from build123d import *

# Parameters (mm, degrees)
F0_W      = 82.55
F0_H      = 82.55
F1_DEPTH  = 38.1
F2_W      = 82.55
F2_H      = 82.55
F2_W_2    = 13.9428069815
F2_H_2    = 9.9208420143
F2_W_3    = 8.0439243466
F2_H_3    = 6.4351418987
F2_W_4    = 8.2115095574
F2_H_4    = 6.1912699603
F2_W_5    = 5.6307478808
F2_H_5    = 5.2285513375
F2_W_6    = 10.3230390232
F2_H_6    = 9.3845799565
F2_W_7    = 7.6417308301
F2_H_7    = 7.5076650828
F2_W_8    = 12.3340208083
F2_H_8    = 10.3230387904
F2_W_9    = 7.9098585993
F2_H_9    = 7.5076660141
F2_W_10   = 7.2456169873
F2_H_10   = 6.6790115088
F2_W_11   = 6.5692057833
F2_H_11   = 4.9604205415
F2_W_12   = 14.4120394252
F2_H_12   = 10.4571059346
F2_W_13   = 11.3955624402
F2_H_13   = 10.1889744401
F2_W_14   = 6.7032724619
F2_H_14   = 5.6307483464
F2_W_15   = 5.6307520717
F2_H_15   = 5.3626168519
F3_DEPTH  = 2.54
F4_W      = 82.55
F4_H      = 12.5048903072
F5_DEPTH  = 2.286
F6_W      = 8.554907316
F6_H      = 8.3226170391
F7_DEPTH  = 2.286
F8_W      = 8.5991304368
F8_H      = 7.9995281994
F9_DEPTH  = 2.286
F10_W     = 9.0507952429
F10_H     = 8.4728021175
F11_DEPTH = 2.286
F12_W     = 7.5796225905
F12_H     = 8.1127006561
F13_DEPTH = 2.286
F14_W     = 84.836
F14_H     = 12.5993990594
F15_DEPTH = 2.286
F16_W     = 5.275822799
F16_H     = 8.0181919038
F17_DEPTH = 2.286
F18_W     = 2.1420419216
F18_H     = 8.0181919038
F19_DEPTH = 2.286
F20_W     = 9.7789997235
F20_H     = 7.7714007348
F21_DEPTH = 2.286
F22_W     = 8.092913311
F22_H     = 7.8396778554
F23_DEPTH = 2.286
F24_W     = 7.9482773185
F24_H     = 8.0201905221
F25_DEPTH = 2.286
F26_W     = 84.836
F26_H     = 12.4227774584
F27_DEPTH = 2.286
F28_W     = 5.6573223279
F28_H     = 8.1968121231
F29_DEPTH = 2.286
F30_W     = 2.7038902044
F30_H     = 8.1968121231
F31_DEPTH = 2.286
F32_W     = 11.1818928272
F32_H     = 7.734913379
F33_DEPTH = 2.286
F34_W     = 11.2993712537
F34_H     = 7.8291036189
F35_DEPTH = 2.286
F36_W     = 7.6127404213
F36_H     = 7.734913379
F37_DEPTH = 2.286
F38_W     = 87.122
F38_H     = 10.4137536731
F39_DEPTH = 2.286
F40_W     = 4.9288716123
F40_H     = 9.7913470712
F40_W_2   = 2.5759153068
F41_DEPTH = 2.286
F42_W     = 11.5772541612
F42_H     = 9.7913470712
F43_DEPTH = 2.286
F44_W     = 13.4015749209
F44_H     = 9.7913470712
F45_DEPTH = 2.286
F46_W     = 7.5191628144
F46_H     = 10.4137536731
F47_DEPTH = 2.286
F48_SCALE = 1.5


with BuildPart() as f1:
    # F0 (on Top) → F1 (new body)
    with BuildSketch(Plane.XY):
        Rectangle(F0_W, F0_H)
    extrude(amount=F1_DEPTH)

    # F2 (on face) → F3 (join)
    with BuildSketch(Plane.XY.offset(38.1)):
        Rectangle(F2_W, F2_H)
        with Locations((-21.3224873878, -29.7867883928)):
            Rectangle(F2_W_2, F2_H_2, mode=Mode.SUBTRACT)
        with Locations((-28.6960853264, -13.6989350431)):
            Rectangle(F2_W_3, F2_H_3, mode=Mode.SUBTRACT)
        with Locations((-21.1381489644, -3.0956349801)):
            Rectangle(F2_W_4, F2_H_4, mode=Mode.SUBTRACT)
        with Locations((-8.3181404043, -6.3923679991)):
            Rectangle(F2_W_5, F2_H_5, mode=Mode.SUBTRACT)
        with Locations((2.6081927354, -24.1560377181)):
            Rectangle(F2_W_6, F2_H_6, mode=Mode.SUBTRACT)
        with Locations((17.6235223189, -27.1054795012)):
            Rectangle(F2_W_7, F2_H_7, mode=Mode.SUBTRACT)
        with Locations((11.9257410988, -0.8956852835)):
            Rectangle(F2_W_8, F2_H_8, mode=Mode.SUBTRACT)
        with Locations((34.6498331055, -15.5758508481)):
            Rectangle(F2_W_9, F2_H_9, mode=Mode.SUBTRACT)
        with Locations((-3.6228084937, 3.3395057544)):
            Rectangle(F2_W_10, F2_H_10, mode=Mode.SUBTRACT)
        with Locations((-18.0378840305, 10.7680070214)):
            Rectangle(F2_W_11, F2_H_11, mode=Mode.SUBTRACT)
        with Locations((-25.2439037431, 22.9009296745)):
            Rectangle(F2_W_12, F2_H_12, mode=Mode.SUBTRACT)
        with Locations((-1.5478357673, 24.9119121581)):
            Rectangle(F2_W_13, F2_H_13, mode=Mode.SUBTRACT)
        with Locations((30.6949019432, 10.7680070214)):
            Rectangle(F2_W_14, F2_H_11, mode=Mode.SUBTRACT)
        with Locations((16.6180301458, 21.5602749959)):
            Rectangle(F2_W_14, F2_H_14, mode=Mode.SUBTRACT)
        with Locations((27.87952777, 30.8107910678)):
            Rectangle(F2_W_15, F2_H_15, mode=Mode.SUBTRACT)
    extrude(amount=F3_DEPTH)

    # F4 (on face) → F5 (join)
    with BuildSketch(Plane.YZ.offset(41.275)):
        with Locations((0, 34.3875548464)):
            Rectangle(F4_W, F4_H)
    extrude(amount=F5_DEPTH)

    # F6 (on face) → F7 (join)
    with BuildSketch(Plane.YZ.offset(41.275)):
        with Locations((-36.997546342, 23.9738011733)):
            Rectangle(F6_W, F6_H)
    extrude(amount=F7_DEPTH)

    # F8 (on face) → F9 (join)
    with BuildSketch(Plane.YZ.offset(41.275)):
        with Locations((-15.3713310137, 24.1353455931)):
            Rectangle(F8_W, F8_H)
    extrude(amount=F9_DEPTH)

    # F10 (on face) → F11 (join)
    with BuildSketch(Plane.YZ.offset(41.275)):
        with Locations((10.5762194809, 23.8987086341)):
            Rectangle(F10_W, F10_H)
    extrude(amount=F11_DEPTH)

    # F12 (on face) → F13 (join)
    with BuildSketch(Plane.YZ.offset(41.275)):
        with Locations((37.4851887047, 24.0787593648)):
            Rectangle(F12_W, F12_H)
    extrude(amount=F13_DEPTH)

    # F14 (on face) → F15 (join)
    with BuildSketch(Plane(origin=(0, 41.275, 0), x_dir=(-1, 0, 0), z_dir=(0, 1, 0))):
        with Locations((-1.143, 34.3403004703)):
            Rectangle(F14_W, F14_H)
    extrude(amount=F15_DEPTH)

    # F16 (on face) → F17 (join)
    with BuildSketch(Plane(origin=(0, 41.275, 0), x_dir=(-1, 0, 0), z_dir=(0, 1, 0))):
        with Locations((-40.9230886005, 24.0315049887)):
            Rectangle(F16_W, F16_H)
    extrude(amount=F17_DEPTH)

    # F18 (on face) → F19 (join)
    with BuildSketch(Plane(origin=(0, 41.275, 0), x_dir=(-1, 0, 0), z_dir=(0, 1, 0))):
        with Locations((-37.2141562402, 24.0315049887)):
            Rectangle(F18_W, F18_H)
    extrude(amount=F19_DEPTH)

    # F20 (on face) → F21 (join)
    with BuildSketch(Plane(origin=(0, 41.275, 0), x_dir=(-1, 0, 0), z_dir=(0, 1, 0))):
        with Locations((-16.2686998956, 24.1549005732)):
            Rectangle(F20_W, F20_H)
    extrude(amount=F21_DEPTH)

    # F22 (on face) → F23 (join)
    with BuildSketch(Plane(origin=(0, 41.275, 0), x_dir=(-1, 0, 0), z_dir=(0, 1, 0))):
        with Locations((11.0376609955, 24.1207620129)):
            Rectangle(F22_W, F22_H)
    extrude(amount=F23_DEPTH)

    # F24 (on face) → F25 (join)
    with BuildSketch(Plane(origin=(0, 41.275, 0), x_dir=(-1, 0, 0), z_dir=(0, 1, 0))):
        with Locations((37.3008613408, 24.0305056795)):
            Rectangle(F24_W, F24_H)
    extrude(amount=F25_DEPTH)

    # F26 (on face) → F27 (join)
    with BuildSketch(Plane(origin=(-41.275, 0, 0), x_dir=(0, -1, 0), z_dir=(-1, 0, 0))):
        with Locations((-1.143, 34.4286112708)):
            Rectangle(F26_W, F26_H)
    extrude(amount=F27_DEPTH)

    # F28 (on face) → F29 (join)
    with BuildSketch(Plane(origin=(-41.275, 0, 0), x_dir=(0, -1, 0), z_dir=(-1, 0, 0))):
        with Locations((-40.7323388361, 24.11881648)):
            Rectangle(F28_W, F28_H)
    extrude(amount=F29_DEPTH)

    # F30 (on face) → F31 (join)
    with BuildSketch(Plane(origin=(-41.275, 0, 0), x_dir=(0, -1, 0), z_dir=(-1, 0, 0))):
        with Locations((-36.5517325699, 24.11881648)):
            Rectangle(F30_W, F30_H)
    extrude(amount=F31_DEPTH)

    # F32 (on face) → F33 (join)
    with BuildSketch(Plane(origin=(-41.275, 0, 0), x_dir=(0, -1, 0), z_dir=(-1, 0, 0))):
        with Locations((-16.6591824964, 24.3497658521)):
            Rectangle(F32_W, F32_H)
    extrude(amount=F33_DEPTH)

    # F34 (on face) → F35 (join)
    with BuildSketch(Plane(origin=(-41.275, 0, 0), x_dir=(0, -1, 0), z_dir=(-1, 0, 0))):
        with Locations((10.0554807577, 24.3026707321)):
            Rectangle(F34_W, F34_H)
    extrude(amount=F35_DEPTH)

    # F36 (on face) → F37 (join)
    with BuildSketch(Plane(origin=(-41.275, 0, 0), x_dir=(0, -1, 0), z_dir=(-1, 0, 0))):
        with Locations((37.4686297894, 24.3497658521)):
            Rectangle(F36_W, F36_H)
    extrude(amount=F37_DEPTH)

    # F38 (on face) → F39 (join)
    with BuildSketch(Plane.XZ.offset(41.275)):
        with Locations((0, 35.4331231634)):
            Rectangle(F38_W, F38_H)
    extrude(amount=F39_DEPTH)

    # F40 (on face) → F41 (join)
    with BuildSketch(Plane.XZ.offset(41.275)):
        with Locations((-41.0965641938, 25.3305727912)):
            Rectangle(F40_W, F40_H)
        with Locations((-37.3441707343, 25.3305727912)):
            Rectangle(F40_W_2, F40_H)
    extrude(amount=F41_DEPTH)

    # F42 (on face) → F43 (join)
    with BuildSketch(Plane.XZ.offset(41.275)):
        with Locations((-18.2089535519, 25.3305727912)):
            Rectangle(F42_W, F42_H)
    extrude(amount=F43_DEPTH)

    # F44 (on face) → F45 (join)
    with BuildSketch(Plane.XZ.offset(41.275)):
        with Locations((13.1122844759, 25.3305727912)):
            Rectangle(F44_W, F44_H)
    extrude(amount=F45_DEPTH)

    # F46 (on face) → F47 (join)
    with BuildSketch(Plane.XZ.offset(41.275)):
        with Locations((39.8014185928, 25.0193694903)):
            Rectangle(F46_W, F46_H)
    extrude(amount=F47_DEPTH)


with BuildPart() as f1_1:
    # F48: moved
    add(f1.part.scale(F48_SCALE))


solid = f1_1.part
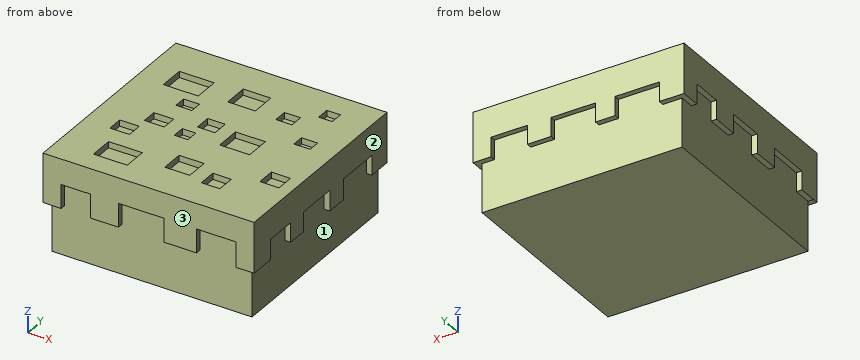
Could you check a few things on this model? Use its own coordinates, in mm. Face numbers are marked on the shaded views. Give positions to 0.01 mm unless a question says otherwise; leave off trailing zeros. Order: outer loops, then holes, each group sorted by start corner. A loop starts at its lowest first (then second) coordinate and runs counter-clockwise, first axis right, second up.
Item 1: If we section it at A-A, the plane x = -57: Write out the boundary of the cut face in (y, z), plus the area to 3 significant figures.
Item 2: If we section it at B-B, the plane y = 40: Write out the boundary of the cut face in (x, z).
Item 3: I'm going to push flat-ended pins straight in: pin 1 (3.5 mm diameter, centred on x = 48, y = 17.5, fed in from +Z); pin 2 (1.7 mm diameter, centred on x = 22.5, y = 63.5, fed in from -Z); pin 3 (10 mm diameter, centred on y = 43, z = 10.5, fed in from +X). Where does each tip first touch, or does it pass through?
Item 4: If we section it at D-D, the plane z = 22.5: Write out the boundary of the cut face in (x, y), plus the area to 3 significant figures.
Item 5: I need wall thicknesses on line 1 (X direction, y = -29.5, z = 10); line 2 (Y direction, x = -6, z = 45). Which ranges of each line are inside material? Lowest first, please.
Item 6: If we section it at C-C, the plane x = 44: Write out the boundary of the cut face in (y, z), plus the area to 3 significant figures.
Item 7: If we mould it in two halves opening along Y, with no side actions, what happens to the marked faces 1, 2 and 3? For each: pulls with the +Y half, pulls with the -Y half, needs draft (parallel to the pull), parting line crosses it, or undercut.
Values:
1. outline: (-65.34, 30.65) - (-61.91, 30.65) - (-61.91, 0) - (61.91, 0) - (61.91, 30.03) - (65.34, 30.03) - (65.34, 60.96) - (-65.34, 60.96) - close
1. area: 7,760 mm2
2. outline: (-65.34, 42.33) - (-61.91, 42.33) - (-61.91, 0) - (61.91, 0) - (61.91, 42.2) - (65.34, 42.2) - (65.34, 60.96) - (6.22, 60.96) - (6.22, 57.15) - (-10.87, 57.15) - (-10.87, 60.96) - (-27.06, 60.96) - (-27.06, 57.15) - (-48.67, 57.15) - (-48.67, 60.96) - (-65.34, 60.96) - close
3. pin 1: stops at z = 57.15
3. pin 2: stops at z = 30.4
3. pin 3: stops at x = 61.91
4. outline: (-61.91, -61.91) - (61.91, -61.91) - (61.91, 61.91) - (-61.91, 61.91) - close
4. area: 15,300 mm2
5. line 1: x = -61.91 to 61.91
5. line 2: y = -61.91 to 65.34
6. outline: (-65.34, 45.34) - (-61.91, 45.34) - (-61.91, 0) - (61.91, 0) - (61.91, 42.06) - (65.34, 42.06) - (65.34, 60.96) - (50.24, 60.96) - (50.24, 57.15) - (42.19, 57.15) - (42.19, 60.96) - (19.87, 60.96) - (19.87, 57.15) - (12.43, 57.15) - (12.43, 60.96) - (-65.34, 60.96) - close
6. area: 7,610 mm2
7. face 1: undercut
7. face 2: needs draft
7. face 3: pulls with the -Y half
